Input: part model. Units: mm. Frame: model coordinates. Face numbers are marked on the shaded views. A direction names the side the tool comes from. Coordinates: 2 decimals unless noted, no trailing zeros. Loops run counter-clockwise (first coordinate to the right, second up) from the corner with the lowest first, then second, coordinate; pieces in that order, holes last. Notation, with made-up numbers: (30, 2.25) - (60, 2.25) arc R23 ccw to (60, 21.25) - close; hole circle Ø2 at (41.5, 57). An arc over 180 degrees is marked (long way). Use a Markdown table: item, result. Add a question column.
1. Draft query along Y for the marked faces 3, 4 and 5. Return one class per face: released by +Y, released by -Y, zero draft, split by the parting line, or undercut.
2. Contact query for flat-ended pins moving along their axis: P1, Ø1, axis at x = 3, y = 2, coming from the -Z side; P2, Ø3, axis at x = 0, z = 0.5, coming from the -Y side; P3, Ø1.4, axis at x = 1, y = 0.5, coming from the +Z side. Output: stop coordinate, or through.
3. Section query B-B on z = -1.25. Return the cut outline in (x, y).
4. Access query for the marked faces 1 and 2. Directions: +Z, -Z, +X, -X, +Y, -Y. A direction counts if a zero-diameter tool reaches every point of the face in a straight line with its end or side. Return the directions, or none.
5. Ray query, L1, parallel to X at y = 0.75, z = -3.25; L2, parallel to Z at x = -1, y = 2.25; L3, parallel to Z at x = -0.25, y = -2.5. Return the intervals inside material, ascending. Write a range as [from, to].
6. Section query C-C on z = 1. Return the cut outline in (x, y) (3 decimals).
7. Section query A-A on z = 3.5. Return the cut outline in (x, y) (3 decimals), then the cut area to 3 significant figures.
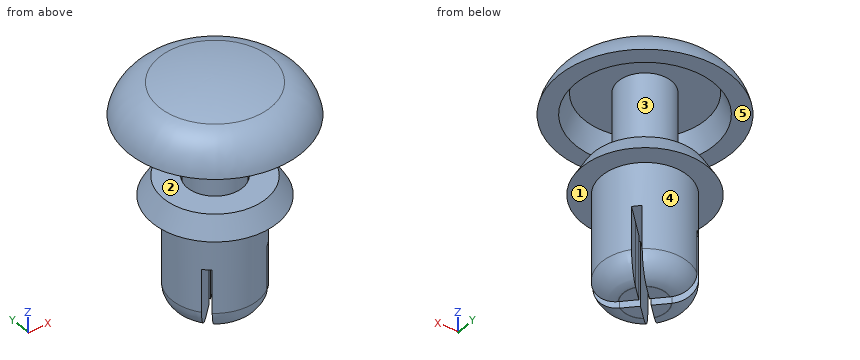
Autodesk Inventor part; units mm, degrees
ref_plane "YZ Plane" through (0, 0, 0) normal (1, 0, 0) x (0, 1, 0)
ref_plane "XZ Plane" through (0, 0, 0) normal (0, 1, 0) x (-1, 0, 0)
ref_plane "XY Plane" through (0, 0, 0) normal (0, 0, 1) x (1, 0, 0)
sketch "Sketch1" plane through (0, 0, 0) normal (0, 1, 0) x (-1, 0, 0)
  arc A0 (2.5786, 4.3289) -> (0, 4.6354) centre (0, -6.3646) ccw
  arc A1 (4, 2.8354) -> (2.5786, 4.3289) centre (2.1332, 2.4819) ccw
  line L0 (4, 2.8354) -> (3.2, 2.8354)
  line L1 (3.2, 2.8354) -> (2.8, 3.8354)
  line L2 (2.8, 3.8354) -> (1.225, 3.8354)
  line L3 (1.225, 3.8354) -> (1.225, -0.9)
  line L4 (1.225, -0.9) -> (1.275, -0.9)
  line L5 (1.275, -0.9) -> (1.275, 0)
  line L6 (1.275, 0) -> (2.3804, 0)
  line L7 (2.3804, 0) -> (2.9, -0.9)
  line L8 (2.9, -0.9) -> (1.99, -0.9)
  line L9 (1.275, -1.5) -> (1.225, -1.5)
  arc A2 (2.5786, 4.3289) -> (0, 4.6354) centre (0, -6.3646) ccw
  arc A3 (4, 2.8354) -> (2.5786, 4.3289) centre (2.1332, 2.4819) ccw
  line L10 (4, 2.8354) -> (3.2, 2.8354)
  line L11 (3.2, 2.8354) -> (2.8, 3.8354)
  line L12 (2.8, 3.8354) -> (1.225, 3.8354)
  line L13 (1.225, 3.8354) -> (1.225, -0.9)
  line L14 (1.225, -0.9) -> (1.275, -0.9)
  line L15 (1.275, -0.9) -> (1.275, 0)
  line L16 (1.275, 0) -> (2.3804, 0)
  line L17 (2.3804, 0) -> (2.9, -0.9)
  line L18 (2.9, -0.9) -> (2, -0.9)
  line L19 (1.275, -1.5) -> (1.225, -1.5)
  line L20 (1.99, -4.9) -> (1.99, -0.9)
  spline S0 degree 3 poles (1.99, -4.9) (1.99, -5.0231) (1.9611, -5.1679) (1.8666, -5.3956) (1.7841, -5.5186) (1.6089, -5.6933) (1.4849, -5.7757) (1.2538, -5.871) (1.1056, -5.9) (0.9798, -5.9) knots -0.250479 -0.250479 -0.250479 -0.250479 -0.213555 -0.213555 -0.176537 -0.176537 -0.139311 -0.139311 -0.101565 -0.101565 -0.101565 -0.101565
  line L21 (0, -5.9) -> (1, -5.9)
  line L22 (0, 4.6354) -> (0, -5.9)
  point P0 (0, 0)
  point P1 (0, 0)
revolve "Revolution1" add sketch "Sketch1" angle 360 about axis through (0, 0, 4.6354) along (0, 0, -1)
sketch "Sketch2" plane through (0, 0, -5.9) normal (0, 0, -1) x (-1, 0, 0)
  line L0 (0.8343, -0.5514) -> (0.2829, 0)
  line L1 (0.2829, 0) -> (0.8343, 0.5514)
  arc A0 (0.8343, -0.5514) -> (0.8343, 0.5514) centre (0, 0) ccw
  line L2 (-0.5514, -0.8343) -> (0, -0.2829)
  line L3 (0, -0.2829) -> (1.2657, -1.5486)
  arc A1 (-0.5514, -0.8343) -> (0.5514, -0.8343) centre (0, 0) ccw
  line L4 (-0.2829, 0) -> (-1.5486, -1.2657)
  arc A2 (-0.8343, 0.5514) -> (-0.8343, -0.5514) centre (0, 0) ccw
  line L5 (-0.8343, 0.5514) -> (-0.2829, 0)
  line L6 (0, 0.2829) -> (-1.2657, 1.5485)
  arc A3 (0.5514, 0.8343) -> (-0.5514, 0.8343) centre (0, 0) ccw
  line L7 (1.2657, 1.5486) -> (0, 0.2829)
  circle A4 centre (0, 0) radius 2.9
  line L8 (-1.2657, -1.5485) -> (-0.5514, -0.8343)
  line L9 (-1.5485, 1.2657) -> (-0.8343, 0.5514)
  line L10 (1.5485, -1.2656) -> (0.8343, -0.5514)
  line L11 (0.8343, 0.5514) -> (1.5485, 1.2657)
  arc A5 (1.2656, -1.5485) -> (1.5485, -1.2656) centre (0, 0) ccw
  arc A6 (-1.5485, -1.2656) -> (-1.2656, -1.5485) centre (0, 0) ccw
  arc A7 (1.5485, 1.2657) -> (1.2657, 1.5485) centre (0, 0) ccw
  arc A8 (-1.2656, 1.5485) -> (-1.5485, 1.2656) centre (0, 0) ccw
  point P0 (0, 0)
extrude "Extrusion1" cut sketch "Sketch2" against normal blind 3 contours L10 A5 L3 L2 L8 A6 L4 L5 L9 A8 L6 L7 A7 L11 L1 L0
properties part number "11-6001" material "Polystyrene, High Impact"
Resolved:
| question | item | result |
|---|---|---|
| 1 | face 3 | undercut |
| 1 | face 4 | split by the parting line |
| 1 | face 5 | zero draft |
| 2 | P1 | z = 2.84 |
| 2 | P2 | y = -2.9 |
| 2 | P3 | z = 4.63 |
| 3 | outline | circle Ø3.98 at (0, 0) |
| 4 | face 1 | -Z |
| 4 | face 2 | none |
| 5 | L1 | [-1.84, -1.03], [-0.47, 0.47], [1.03, 1.84] |
| 5 | L2 | [-0.9, -0.14], [3.84, 4.36] |
| 5 | L3 | [-0.9, -0.23], [3.84, 4.34] |
| 6 | outline | circle Ø2.45 at (0, 0) |
| 7 | outline | circle Ø7.475 at (0, 0); circle Ø2.45 at (0, 0); hole circle Ø5.868 at (0, 0) |
| 7 | area | 21.5 mm² |
